For this review, take the finished solid that the model builds, in its own axes (mm). Round coordinates to 2 decimals unless told otherwise and drop trailing zeros. Write each loop counter-clockwise with the first axis right and the second up, starting at its lowest first coordinate (ties: lowest second). Pieces come first, ordered by that corner, then holes. Notation, with made-up numbers: (-20.75, 14) -> (8.25, 14) arc R22 ccw to (8.25, 53) -> close; hole circle Ø3 at (37.5, 78). An arc over 180 degrees is marked (long way). Write each question's results on one line, items separated by ' | '. Start each with the question number.
Item 1: Add section D-D (z = -33). State the section outline as (x, y) points, plus the area to 3 significant figures.
Item 2: Clearance check with flat-ended pins moving along their axes: pin 1 (1.5 mm diameter, centred on y = 2, z = -93, fed in from +X); pin 2 (1.5 mm diameter, centred on x = 69.5, y = 1.5, fed in from -Z); pin 3 (1.5 mm diameter, centred on y = 4.5, z = -66.5, fed in from +X). State where each tip first meets the part, or that it passes through.
Item 3: To check wall thickness, follow line 1 along Z through (x, y) = (22.5, 1.8); line 2 along Z through (x, y) = (100, 1.15); line 3 along Z through (x, y) = (59, 4). State the ranges of each line that lie inside material, in increasing order.
Item 4: Add section C-C (x = 78). State the section outline as (y, z) points, plus the area to 3 significant figures.
Item 5: Add section A-A (z = -15). Count the separate pieces of the cut face and the enclosed holes in it, plus the area to 3 significant figures.
from build123d import *

# Parameters (mm, degrees)
SKETCH1_R           = 15
SKETCH1_R_2         = 7.396823718
BOSS_EXTRUDE1_DEPTH = 5


with BuildPart() as part:
    # Sketch1 → Boss-Extrude1 (new body)
    with BuildSketch(Plane(origin=(0, 0, 0), x_dir=(1, 0, 0), z_dir=(0, 1, 0))):
        with BuildLine():
            Line((155, 0), (155, 20))
            ThreePointArc((155, 20), (152.071067812, 27.071067812), (145, 30))
            Line((145, 30), (130.631756617, 30))
            ThreePointArc((130.631756617, 30), (125.186785887, 31.612372579), (121.497679457, 35.929541251))
            ThreePointArc((121.497679457, 35.929541251), (99.953355799, 63.858544428), (68.011045902, 78.821028806))
            ThreePointArc((68.011045902, 78.821028806), (62.257599178, 82.292315938), (60, 88.621236029))
            Line((60, 88.621236029), (60, 100))
            ThreePointArc((60, 100), (57.071067812, 107.071067812), (50, 110))
            Line((50, 110), (10, 110))
            ThreePointArc((10, 110), (2.928932188, 107.071067812), (0, 100))
            Line((0, 100), (0, 0))
            Line((0, 0), (155, 0))
        make_face()
        with Locations((30, 90)):
            Circle(SKETCH1_R, mode=Mode.SUBTRACT)
        with Locations((20, 15)):
            Circle(SKETCH1_R_2, mode=Mode.SUBTRACT)
        with Locations((40, 15)):
            Circle(SKETCH1_R_2, mode=Mode.SUBTRACT)
        with Locations((60, 15)):
            Circle(SKETCH1_R_2, mode=Mode.SUBTRACT)
        with Locations((80, 15)):
            Circle(SKETCH1_R_2, mode=Mode.SUBTRACT)
        with Locations((100, 15)):
            Circle(SKETCH1_R_2, mode=Mode.SUBTRACT)
        with Locations((120, 15)):
            Circle(SKETCH1_R_2, mode=Mode.SUBTRACT)
        with Locations((140, 15)):
            Circle(SKETCH1_R_2, mode=Mode.SUBTRACT)
        with BuildLine():
            ThreePointArc((30, 60), (22.928932188, 57.071067812), (20, 50))
            Line((20, 50), (20, 30))
            Line((20, 30), (101.830075275, 30))
            ThreePointArc((101.830075275, 30), (81.724911294, 51.898267594), (53.122224807, 60))
            Line((53.122224807, 60), (30, 60))
        make_face(mode=Mode.SUBTRACT)
    extrude(amount=BOSS_EXTRUDE1_DEPTH)


solid = part.part
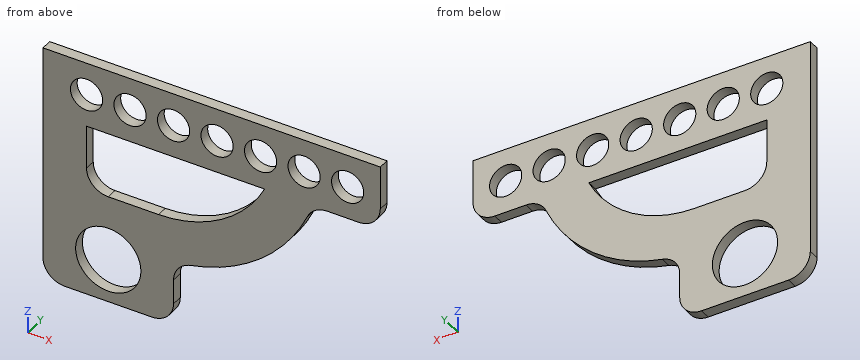
Responses:
1) outline: (0, 0) -> (20, 0) -> (20, 5) -> (0, 5) -> close; (100.2, 0) -> (123.49, 0) -> (123.49, 5) -> (100.2, 5) -> close | area: 216 mm^2
2) pin 1: stops at x = 60 | pin 2: stops at z = -78.67 | pin 3: stops at x = 97.49
3) line 1: z = -110 to -102.99, -77.01 to -56.61, -30 to -21.96, -8.04 to 0 | line 2: z = -63.82 to -33.34, -30 to -22.4, -7.6 to 0 | line 3: z = -104.36 to -59.68, -30 to -22.33, -7.67 to 0
4) outline: (0, -76.06) -> (5, -76.06) -> (5, -54) -> (0, -54) -> close; (0, -30) -> (5, -30) -> (5, -22.12) -> (0, -22.12) -> close; (0, -7.88) -> (5, -7.88) -> (5, 0) -> (0, 0) -> close | area: 189 mm^2
5) separate pieces: 8 | enclosed holes: 0 | area: 257 mm^2
